The listing builds one solid part. Answer for the finished solid, in the listing's coordinates (mm). A direction names the side the tool comes from. Give positions to 0.01 mm unless a question says otherwise; leave off trailing zeros. Order: outer loops, then holes, each group sorted by start corner. A loop starts at its lowest first (then second) coordinate and runs counter-clockwise, first axis right, second up. Notation, with made-up numbers: (54.5, 54) - (93.5, 54) arc R17 cw to (93.5, 84) - close; hole circle Ø2 at (-29.75, 64). An arc over 180 degrees is marked (long way). Answer in a Markdown table with one row per item.
Autodesk Inventor part; units mm, degrees
ref_plane "YZ Plane" through (0, 0, 0) normal (1, 0, 0) x (0, 1, 0)
ref_plane "XZ Plane" through (0, 0, 0) normal (0, 1, 0) x (-1, 0, 0)
ref_plane "XY Plane" through (0, 0, 0) normal (0, 0, 1) x (1, 0, 0)
sketch "Sketch14" plane through (0, 0, 0) normal (0, 0, 1) x (1, 0, 0)
  line L0 (-34.54, -49.54) -> (34.54, -49.54)
  line L1 (34.54, -49.54) -> (34.54, 49.54)
  line L2 (34.54, 49.54) -> (-34.54, 49.54)
  line L3 (-34.54, 49.54) -> (-34.54, -49.54)
  line L4 (-34.54, -49.54) -> (34.54, 49.54) construction
  line L5 (34.54, -49.54) -> (-34.54, 49.54) construction
  point P0 (0, 0)
  dimension "d66" = 69.08
  dimension "d67" = 99.08
extrude "Extrusion9" add sketch "Sketch14" against normal blind 2.54
sketch "Sketch15" plane through (0, 0, 0) normal (0, 0, 1) x (1, 0, 0)
  line L0 (-34.54, -49.54) -> (-34.54, 49.54)
  line L1 (34.54, 49.54) -> (34.54, -49.54)
  line L2 (-34.54, -49.54) -> (34.54, -49.54)
  line L3 (34.54, -49.54) -> (34.54, 49.54)
  line L4 (34.54, 49.54) -> (-34.54, 49.54)
  line L5 (-34.54, 49.54) -> (-34.54, -49.54)
  line L6 (-32, -47) -> (32, -47)
  line L7 (32, -47) -> (32, 47)
  line L8 (32, 47) -> (-32, 47)
  line L9 (-32, 47) -> (-32, -47)
  line L10 (-32, -47) -> (32, 47) construction
  line L11 (32, -47) -> (-32, 47) construction
  point P0 (0, 0)
  point P1 (34.54, -49.54)
  dimension "d70" = 64
  dimension "d71" = 94
extrude "Extrusion10" add sketch "Sketch15" along normal blind 34
sketch "Sketch16" plane through (0, 0, 34) normal (0, 0, 1) x (1, 0, 0)
  line L0 (-34.54, -49.54) -> (-34.54, 49.54)
  line L1 (34.54, 49.54) -> (34.54, -49.54)
  line L2 (-34.54, -49.54) -> (34.54, -49.54)
  line L3 (34.54, -49.54) -> (34.54, 49.54)
  line L4 (34.54, 49.54) -> (-34.54, 49.54)
  line L5 (-34.54, 49.54) -> (-34.54, -49.54)
  point P0 (0, 0)
  point P1 (34.54, -49.54)
extrude "Extrusion11" add sketch "Sketch16" along normal blind 2.54
sketch "Sketch17" plane through (-34.54, 49.54, -2.54) normal (0, 1, 0) x (1, 0, 0)
  line L0 (66.54, -2.54) -> (66.54, -36.54)
  line L1 (2.54, -36.54) -> (66.54, -36.54)
  line L2 (2.54, -2.54) -> (2.54, -36.54)
  line L3 (66.54, -2.54) -> (2.54, -2.54)
  line L4 (2.54, -36.54) -> (66.54, -36.54)
  line L5 (66.54, -36.54) -> (66.54, -2.54)
  line L6 (66.54, -2.54) -> (2.54, -2.54)
  line L7 (2.54, -2.54) -> (2.54, -36.54)
  point P0 (34.54, -2.54)
extrude "Extrusion12" cut sketch "Sketch17" against normal blind 2.54
sketch "Sketch18" plane through (34.54, -49.54, -2.54) normal (1, 0, 0) x (0, 0, -1)
  line L0 (-2.54, 2.54) -> (-2.54, 99.08)
  line L1 (-36.54, 99.08) -> (-36.54, 2.54)
  line L2 (-2.54, 2.54) -> (-36.54, 2.54)
  line L3 (-21.54, 7.54) -> (-5.54, 7.54)
  line L4 (-5.54, 7.54) -> (-5.54, 67.54)
  line L5 (-5.54, 67.54) -> (-21.54, 67.54)
  line L6 (-21.54, 67.54) -> (-21.54, 7.54)
  line L7 (-21.54, 7.54) -> (-5.54, 67.54) construction
  line L8 (-5.54, 7.54) -> (-21.54, 67.54) construction
  line L9 (-39.08, 0) -> (-39.08, 99.08)
  point P0 (-2.54, 49.54)
  point P1 (-13.54, 37.54)
  dimension "d78" = 5
  dimension "d79" = 3
  dimension "d80" = 15
  dimension "d81" = 65
extrude "Extrusion13" cut sketch "Sketch18" against normal blind 2.54
sketch "Sketch19" plane through (0, 0, -2.54) normal (0, 0, -1) x (-1, 0, 0)
  line L0 (-25.4, -25.4) -> (25.4, -25.4) construction
  line L1 (25.4, -25.4) -> (25.4, 25.4) construction
  line L2 (25.4, 25.4) -> (-25.4, 25.4) construction
  line L3 (-25.4, 25.4) -> (-25.4, -25.4) construction
  line L4 (-25.4, -25.4) -> (25.4, 25.4) construction
  line L5 (25.4, -25.4) -> (-25.4, 25.4) construction
  point P0 (0, 0)
  dimension "d84" = 50.8
  dimension "d85" = 50.8
hole "Hole3" at (25.4, 25.4, -2.54) at (-25.4, 25.4, -2.54) at (-25.4, -25.4, -2.54) at (25.4, -25.4, -2.54) direction (0, 0, 1) diameter 3.81 end through all
sketch "Sketch22" plane through (0, 0, 36.54) normal (0, 0, 1) x (1, 0, 0)
  circle A0 centre (-25.4, 25.4) radius 1.905
  circle A1 centre (25.4, 25.4) radius 1.905
  circle A2 centre (25.4, -25.4) radius 1.905
  circle A3 centre (-25.4, -25.4) radius 1.905
  point P0 (0, 0)
hole "Hole4" at (-25.4, 25.4, 36.54) at (25.4, 25.4, 36.54) at (25.4, -25.4, 36.54) at (-25.4, -25.4, 36.54) direction (0, 0, -1) diameter 7.62 depth 2.54
equation "\"d66\" = piBoxExteriorWidth"
equation "\"d67\" = piBoxExteriorLength"
equation "\"d68\" = piBoxWallThickness"
equation "\"d70\" = piBoxInteriorWidth"
equation "\"d71\" = piBoxInteriorLength"
equation "\"d72\" = piBoxInteriorHeight"
equation "\"d74\" = piBoxWallThickness"
equation "\"d76\" = piBoxWallThickness"
equation "\"d82\" = piBoxWallThickness"
equation "\"piBoxInteriorLength\" = 94"
equation "\"piBoxInteriorWidth\" = 64"
equation "\"piBoxInteriorHeight\" = 34"
equation "\"piBoxThickness\" = 3.175"
equation "\"piBoxWallThickness\" = 2.54"
equation "\"piBoxExteriorLength\" = piBoxInteriorLength + 2 * piBoxWallThickness"
equation "\"piBoxExteriorHeight\" = piBoxInteriorHeight + piBoxWallThickness"
equation "\"piBoxExteriorWidth\" = piBoxInteriorWidth + 2 * piBoxWallThickness"
properties part number "piCaseAttachesToTripodClamp"
Item 1: Each of these flat-tipped pins is pushed along its axis until it touches: P1, Ø2.5, axis at x = 25.4, y = 25.4, coming from the +Z side; P2, Ø17, axis at x = -11, z = 20, coming from the +Y side; P3, Ø5, axis at x = -25.4, y = -25.4, coming from the +Z side. Where does it stop, or does it pass through?
Answer block:
| item | result |
|---|---|
| P1 | through |
| P2 | y = -47 |
| P3 | z = 0 |
Item 2: Find section C-C on z = 24. Write down the section's boundary in (x, y), then the cut area to 3 significant figures.
Answer block:
| item | result |
|---|---|
| outline | (-34.54, -49.54) - (34.54, -49.54) - (34.54, 49.54) - (32, 49.54) - (32, -47) - (-32, -47) - (-32, 49.54) - (-34.54, 49.54) - close |
| area | 666 mm² |
Item 3: Find section D-D on x = -10.5. Write down the section's boundary in (y, z).
Answer block:
| item | result |
|---|---|
| outline | (-49.54, -2.54) - (49.54, -2.54) - (49.54, 0) - (-47, 0) - (-47, 34) - (49.54, 34) - (49.54, 36.54) - (-49.54, 36.54) - close |
Item 4: Determine the mould class of faces 6 (the face through (-25.484, 23.497, -1.252)), 7 (the face through (0, -47, 17)), 8 (the face through (0, -49.54, 17)), 9 (the face through (33, 18, 11)) for opening direction Y: pulls with the +Y half, pulls with the -Y half, needs draft (parallel to the pull), parting line crosses it, or undercut.
Answer block:
| item | result |
|---|---|
| face 6 | undercut |
| face 7 | pulls with the +Y half |
| face 8 | pulls with the -Y half |
| face 9 | undercut |
Item 5: Find section B-B on y = 40. Write down the section's boundary in (x, z), then the cut area to 3 significant figures.
Answer block:
| item | result |
|---|---|
| outline | (-34.54, -2.54) - (34.54, -2.54) - (34.54, 36.54) - (-34.54, 36.54) - close; hole (-32, 0) - (32, 0) - (32, 34) - (-32, 34) - close |
| area | 524 mm² |
Item 6: Which of the six approach directions +Z, -Z, +X, -X, +Y, -Y give full straight-line access (tool end or side, diameter ignored) to faces 1 (the face through (25.316, -27.303, -1.252)), 2 (the face through (27.72, 28.42, 35.25)), 3 (the face through (-32, 2, 17)), 4 (the face through (33, -12, 3)), 5 (the face through (34.54, 1, 21))?
Answer block:
| item | result |
|---|---|
| face 1 | +Z, -Z |
| face 2 | +Z |
| face 3 | +Y |
| face 4 | +X |
| face 5 | +Z, -Z, +X, +Y, -Y |
Item 7: Consider line 1 (X direction, y = 25.4, z = -1.15) (3 decimals); line 2 (Y direction, x = 25.4, z = -1.1) (3 decimals); line 3 (Y direction, x = -25.4, z = 35.15). Determine where each line is inside the solid, lowest interval first.
Answer block:
| item | result |
|---|---|
| line 1 | -34.54 to -27.305, -23.495 to 23.495, 27.305 to 34.54 |
| line 2 | -49.54 to -27.305, -23.495 to 23.495, 27.305 to 49.54 |
| line 3 | -49.54 to -29.21, -21.59 to 21.59, 29.21 to 49.54 |
Item 8: Find section A-A on y = -25.4. Write down the section's boundary in (x, z) (3 decimals).
Answer block:
| item | result |
|---|---|
| outline | (-34.54, -2.54) - (-27.305, -2.54) - (-27.305, 0) - (-32, 0) - (-32, 34) - (-29.21, 34) - (-29.21, 36.54) - (-34.54, 36.54) - close; (-23.495, -2.54) - (23.495, -2.54) - (23.495, 0) - (-23.495, 0) - close; (-21.59, 34) - (21.59, 34) - (21.59, 36.54) - (-21.59, 36.54) - close; (27.305, -2.54) - (34.54, -2.54) - (34.54, 3) - (32, 3) - (32, 0) - (27.305, 0) - close; (29.21, 34) - (32, 34) - (32, 19) - (34.54, 19) - (34.54, 36.54) - (29.21, 36.54) - close |
